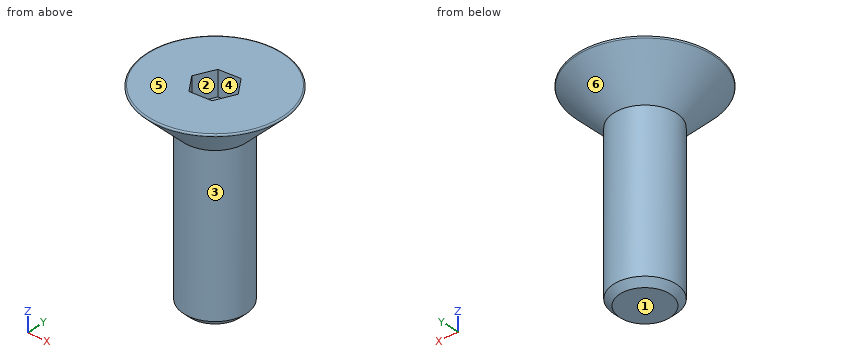
Autodesk Inventor part; units mm, degrees
ref_plane "YZ Plane" through (0, 0, 0) normal (1, 0, 0) x (0, 1, 0)
ref_plane "XZ Plane" through (0, 0, 0) normal (0, 1, 0) x (-1, 0, 0)
ref_plane "XY Plane" through (0, 0, 0) normal (0, 0, 1) x (1, 0, 0)
sketch "Sketch1" plane through (0, 0, 0) normal (0, 0, 1) x (1, 0, 0)
  circle A0 centre (0, 0) radius 2.5
  dimension "Diameter" = 5
extrude "Extrusion1" add sketch "Sketch1" along normal blind 12.9
sketch "Sketch2" plane through (0, 0, 12.9) normal (0, 0, 1) x (1, 0, 0)
  circle A0 centre (0, 0) radius 2.5
extrude "Extrusion2" add sketch "Sketch2" along normal blind 3.1 draft 45
sketch "Sketch3" plane through (0, 0, 16) normal (0, 0, 1) x (1, 0, 0)
  circle A0 centre (0, 0) radius 5.6
  circle A1 centre (0, 0) radius 1.7321 construction
  line L0 (0.725, 1.573) -> (1.7248, 0.1586)
  line L1 (1.7248, 0.1586) -> (0.9997, -1.4144)
  line L2 (0.9997, -1.4144) -> (-0.725, -1.573)
  line L3 (-0.725, -1.573) -> (-1.7248, -0.1586)
  line L4 (-1.7248, -0.1586) -> (-0.9997, 1.4144)
  line L5 (-0.9997, 1.4144) -> (0.725, 1.573)
  dimension "Hex_Width" = 3
extrude "Extrusion3" cut sketch "Sketch3" against normal blind 2 contours L0 L1 L2 L3 L4 L5
thread "Thread1"
chamfer "Chamfer2" distance 0.5 angle 45 1 edges at (-2.5, 0, 0)
fillet "Fillet1" radius 0.1 1 edges at (-5.6, 0, 16)
equation "\"d10\" = Thread_Length"
equation "\"d13\" = Chamfer"
equation "\"Thread_Length\" = 12.9"
equation "\"Length\" = 16"
properties part number "SCREW, FLAT HD, P, 12.9, M5X0.8X16MM"
CAD build for the part. Positions are in the model's coordinates, mm. Face numbers are marked on the shaded views. A direction names the side the tool comes from. Coordinates: 2 decimals unless noted, no trailing zeros. Write each loop counter-clockwise with the first axis right and the second up, starting at its lowest first coordinate (ties: lowest second). Pieces come first, ordered by that corner, then holes. Notation, with made-up numbers: (40.25, -14) - (58.25, -14) arc R19 cw to (58.25, -9) - close; hole circle Ø8 at (40.5, 58). An arc over 180 degrees is marked (long way). Use a Markdown table: item, result. Add a question column.
Item 1: Drill centre lines: L1, parallel to Y at x = -0.75, z = 15.25; L2, parallel to Z at x = -0.25, y = 0; L3, parallel to Y at x = -2.25, z = 2. Where is each one in solid material? Low to high. Write a range as from..to.
Item 2: Band-saw the part on C-C, the plane z = 2.25. Give the cut face in (x, y), and give its area (3 significant figures).
Item 3: Mould opens along Y. For the marked faces 4, 5 and 6 say: pulls with the +Y half, pulls with the -Y half, needs draft (parallel to the pull), parting line crosses it, or undercut.
Item 4: 3-axis set-ups, long thin cutter, end or side, ignore diameter. For the marked faces 1, 2 and 3: which of +Z, -Z, +X, -X, +Y, -Y reach the whole face in a straight line?
Item 5: Band-saw the part on B-B, the plane x = 0. Give the cut face in (y, z).
Item 6: Flat gauge pins, fed straight in: pin 1 (2 mm diameter, centred on y = 2, z = 6.5, fed in from -X); pin 2 (2 mm diameter, centred on x = 0.5, z = 2.5, fed in from -Y); pin 3 (5 mm diameter, centred on y = 4, z = 13.5, fed in from +X). Where does each tip first touch, or does it go through?
Item 7: Band-saw the part on A-A, the plane z = 15. Give the cut face in (x, y) (3 decimals), and give its area (3 significant figures).
Numbers:
| question | item | result |
|---|---|---|
| 1 | L1 | -4.79..-1.54, 1.44..4.79 |
| 1 | L2 | 0..14 |
| 1 | L3 | -1.09..1.09 |
| 2 | outline | circle Ø5 at (0, 0) |
| 2 | area | 19.6 mm2 |
| 3 | face 4 | undercut |
| 3 | face 5 | needs draft |
| 3 | face 6 | parting line crosses it |
| 4 | face 1 | -Z, +X, -X, +Y, -Y |
| 4 | face 2 | +Z |
| 4 | face 3 | -Z |
| 5 | outline | (-5.43, 15.83) - (-2.5, 12.9) - (-2.5, 0.5) - (-2, 0) - (2, 0) - (2.5, 0.5) - (2.5, 12.9) - (5.43, 15.83) arc R0.1 ccw to (5.36, 16) - (1.51, 16) - (1.51, 14) - (-1.51, 14) - (-1.51, 16) - (-5.36, 16) arc R0.1 ccw to start |
| 6 | pin 1 | x = -2.29 |
| 6 | pin 2 | y = -2.5 |
| 6 | pin 3 | x = 4.49 |
| 7 | outline | circle Ø9.2 at (0, 0); hole (-1.725, -0.159) - (-0.725, -1.573) - (1, -1.414) - (1.725, 0.159) - (0.725, 1.573) - (-1, 1.414) - close |
| 7 | area | 58.7 mm2 |
